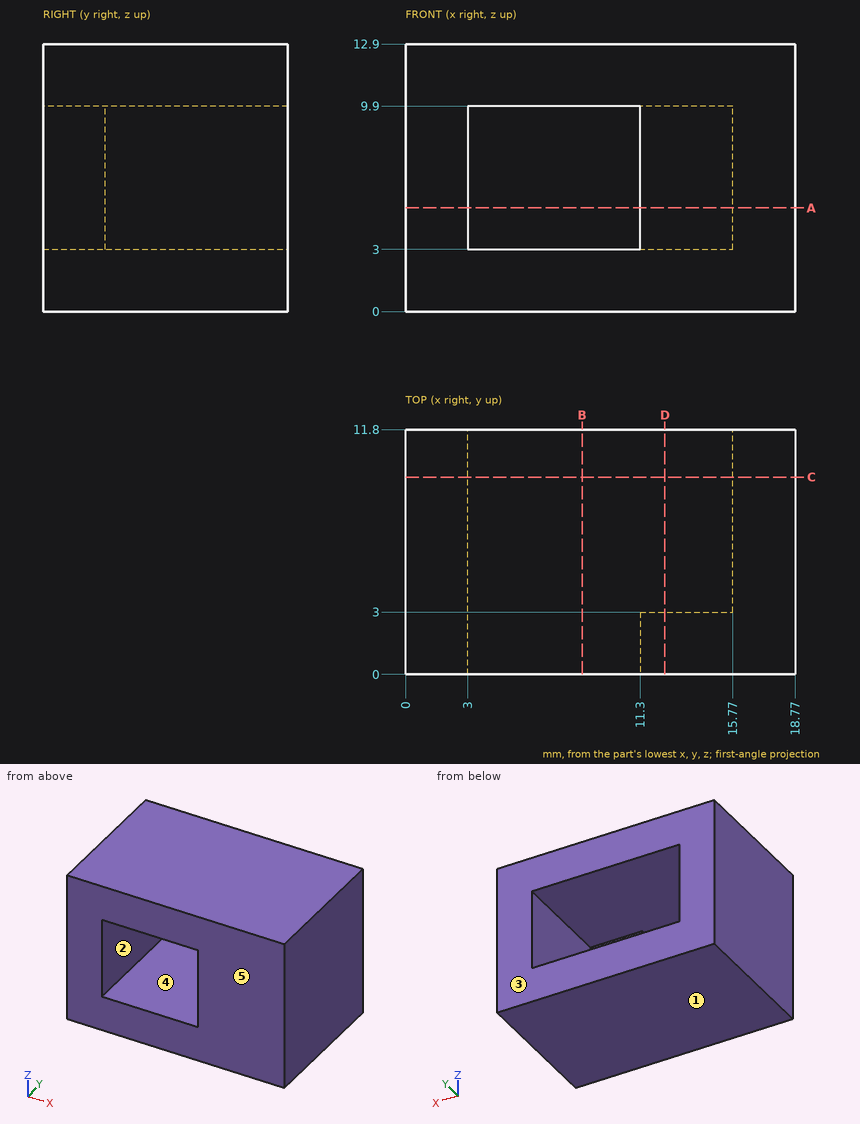
The drawing under review shows one solid part. Ordinate dimensions are in mm from its lowest x, y, z. A direction names the side the tool comes from. Give positions to 0.01 mm unless a question says otherwise; leave off trailing zeros. Write each loop counter-clockwise with the first axis right and the second up, starting at its lowest first coordinate (ties: lowest second). Pieces come first, ordered by that corner, then holes. Notation, with made-up numbers: (56.5, -11.5) -> (71.5, -11.5) arc R32 ccw to (71.5, 25.5) -> close; hole circle Ø6 at (23, 2). An arc over 180 degrees is marked (long way). Answer in a Markdown table with one row per item.
(1) To check wall thickness, follow probe 1 along Z at (x, y) = (10, 3); probe 2 along X at (y, z) = (8.75, 4); probe 3 along Y at (x, z) = (14.25, 6.25). State the ranges of each line that lie inside material, in increasing order.
Results:
| item | result |
|---|---|
| probe 1 | 0 to 3, 9.9 to 12.9 |
| probe 2 | 0 to 3, 15.77 to 18.77 |
| probe 3 | 0 to 3 |
(2) Consider section B-B (x = 8.5). State the section outline as (y, z) points, then the cut area to 3 significant figures.
Results:
| item | result |
|---|---|
| outline | (0, 0) -> (11.8, 0) -> (11.8, 3) -> (0, 3) -> close; (0, 9.9) -> (11.8, 9.9) -> (11.8, 12.9) -> (0, 12.9) -> close |
| area | 70.8 mm2 |
(3) Mouldability with a two-part tool opening along Z and no side actions: class the marked faces 1, 2 and 3 as +Z half, -Z half, draft (parallel to the pull), parting line (faces both ways), or undercut.
Results:
| item | result |
|---|---|
| face 1 | -Z half |
| face 2 | undercut |
| face 3 | draft |
(4) Consider section D-D (x = 12.5). State the section outline as (y, z) points.
Results:
| item | result |
|---|---|
| outline | (0, 0) -> (11.8, 0) -> (11.8, 3) -> (3, 3) -> (3, 9.9) -> (11.8, 9.9) -> (11.8, 12.9) -> (0, 12.9) -> close |
(5) Consider section C-C (y = 9.5). State the section outline as (x, z) points.
Results:
| item | result |
|---|---|
| outline | (0, 0) -> (18.77, 0) -> (18.77, 12.9) -> (0, 12.9) -> close; hole (3, 3) -> (15.77, 3) -> (15.77, 9.9) -> (3, 9.9) -> close |
(6) Clearance check with a flat-ended pin moving along its axis: pin 1 (1.3 mm diameter, centred on x = 13, z = 7, fed in from +Y). State where the tip first meets the part, or that it passes through.
Results:
| item | result |
|---|---|
| pin 1 | y = 3 |
(7) For the marked faces 4 and 5, list the 3-axis set-ups (+Z, -Z, +X, -X, +Y, -Y) from which the entire face can be reached by the end or side of a thin tool; tool diameter is ignored.
Results:
| item | result |
|---|---|
| face 4 | +Y |
| face 5 | +Z, -Z, +X, -X, -Y |
(8) Consider section A-A (z = 5). State the section outline as (x, y) points.
Results:
| item | result |
|---|---|
| outline | (0, 0) -> (3, 0) -> (3, 11.8) -> (0, 11.8) -> close; (11.3, 0) -> (18.77, 0) -> (18.77, 11.8) -> (15.77, 11.8) -> (15.77, 3) -> (11.3, 3) -> close |
